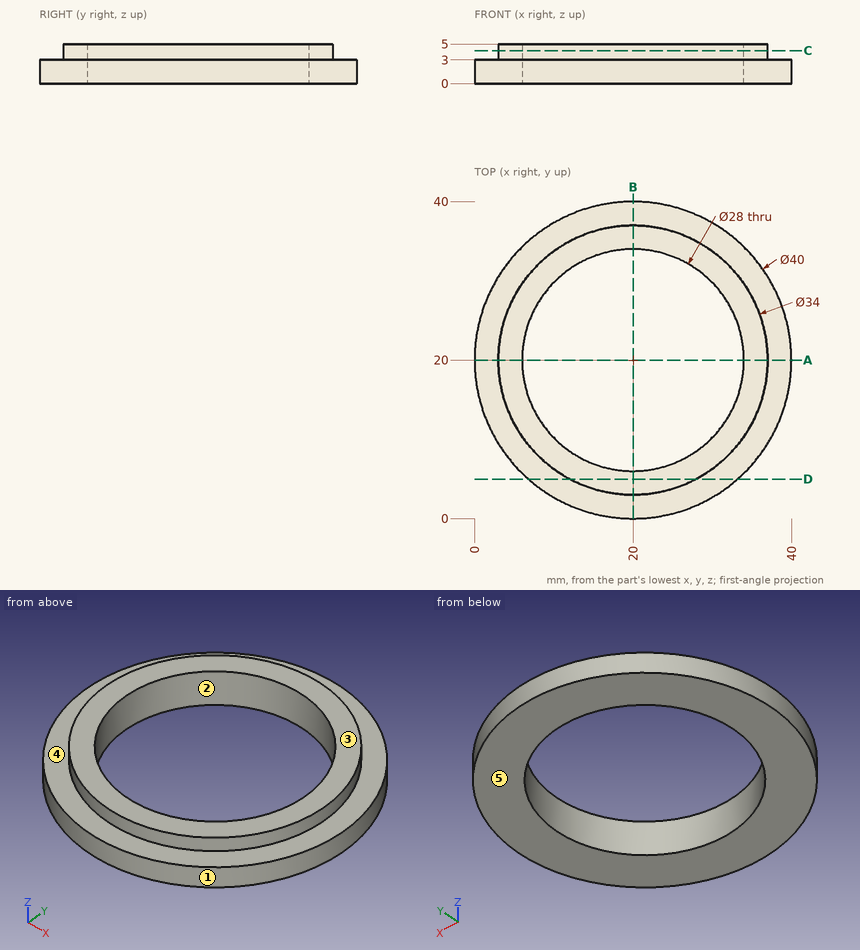
Study the drawing (mm; zero at the part's minimum x, y, z) and answer. A direction names the side the tool comes from. Give positions to 0.01 mm unless a question says otherwise; leave off trailing zeros. Write each loop counter-clockwise with the first axis right and the second up, starting at its lowest first coordinate (ties: lowest second). Pieces come first, ordered by that corner, then holes. Notation, with made-up numbers: (28.5, -25.75) - (35.5, -25.75) arc R36 ccw to (35.5, 9.25) - close; hole circle Ø11 at (29, -33.5). An arc over 180 degrees is marked (long way). Use a Markdown table: item, result.
1. Find the intervals of material crossed by probe 1 along Y at (x, z) = (20, 1.9); probe 2 along Y at (x, z) = (20, 3.75); probe 3 along X at (y, z) = (23.5, 1.6), in increasing order. Write a range as from..to.
Values follow:
| item | result |
|---|---|
| probe 1 | y = 0..6, 34..40 |
| probe 2 | y = 3..6, 34..37 |
| probe 3 | x = 0.31..6.44, 33.56..39.69 |
2. Section C-C on z = 4.15 is taken. Write down the section's boundary in (x, y).
Values follow:
| item | result |
|---|---|
| outline | circle Ø34 at (20, 20); hole circle Ø28 at (20, 20) |
3. For a pull along Y with two mould halves and no side action, classify the marked faces 1, 2 and 3 as released by +Y, released by -Y, zero draft, split by the parting line, or undercut.
Values follow:
| item | result |
|---|---|
| face 1 | split by the parting line |
| face 2 | undercut |
| face 3 | zero draft |
4. A tool of negligible diameter and unlimited length cuts with its end or side. For the marked faces 4 and 5, from which of +Z, -Z, +X, -X, +Y, -Y can it reach the whole face along a straight path? Write none if from no direction.
Values follow:
| item | result |
|---|---|
| face 4 | +Z |
| face 5 | -Z, +X, -X, +Y, -Y |
5. Section D-D on y = 5 is taken. Write down the section's boundary in (x, z).
Values follow:
| item | result |
|---|---|
| outline | (6.77, 0) - (33.23, 0) - (33.23, 3) - (28, 3) - (28, 5) - (12, 5) - (12, 3) - (6.77, 3) - close |
6. Each of these flat-tipped pins is pushed along its axis until it touches: P1, Ø1.5, axis at y = 4.5, z = 3, coming from the -X side; P2, Ø3, axis at y = 34.5, z = 4, coming from the -X side. Where does it stop, or does it pass through?
Values follow:
| item | result |
|---|---|
| P1 | stops at x = 6.49 |
| P2 | stops at x = 5.14 |
7. Section A-A on y = 20 is taken. Write down the section's boundary in (x, z).
Values follow:
| item | result |
|---|---|
| outline | (0, 0) - (6, 0) - (6, 5) - (3, 5) - (3, 3) - (0, 3) - close; (34, 0) - (40, 0) - (40, 3) - (37, 3) - (37, 5) - (34, 5) - close |
